```python
from build123d import *

# Parameters (mm, degrees)
F0_W     = 50.8
F0_H     = 50.8
F1_DEPTH = 38.1
F0_H_2   = 12.7
F0_R     = 2.54
F2_DEPTH = 12.7
F3_SIZE  = 5.08
F4_W     = 25.4
F4_H     = 12.7
F5_DEPTH = 38.1


with BuildPart() as f1:
    # F0 (on Top) → F1 (new body)
    with BuildSketch(Plane.XY):
        with Locations((-76.2, 12.7)):
            Rectangle(F0_W, F0_H)
    extrude(amount=F1_DEPTH)

    # F0 (on Top) → F2 (join)
    with BuildSketch(Plane.XY):
        with Locations((-76.2, -19.05)):
            Rectangle(F0_W, F0_H_2)
        with Locations((-95.25, -19.05)):
            Circle(F0_R, mode=Mode.SUBTRACT)
        with Locations((-57.15, -19.05)):
            Circle(F0_R, mode=Mode.SUBTRACT)
        with Locations((-76.2, 44.45)):
            Rectangle(F0_W, F0_H_2)
        with Locations((-95.25, 44.45)):
            Circle(F0_R, mode=Mode.SUBTRACT)
        with Locations((-57.15, 44.45)):
            Circle(F0_R, mode=Mode.SUBTRACT)
    extrude(amount=F2_DEPTH)

    # F3
    f3_edges = [f1.edges().sort_by_distance(p)[0] for p in [
        (-76.2, 38.1, 38.1),
        (-76.2, -12.7, 38.1),
    ]]
    chamfer(f3_edges, length=F3_SIZE)

    # F4 (on face) → F5 (cut)
    with BuildSketch(Plane.YZ.offset(-50.8)):
        with Locations((12.7, 22.86)):
            Rectangle(F4_W, F4_H)
    extrude(amount=-F5_DEPTH, mode=Mode.SUBTRACT)


solid = f1.part
```
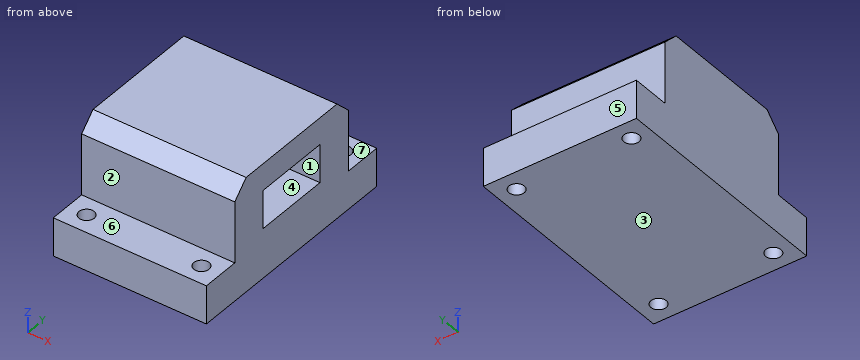
Model file for the job. Use its own axes, mm. Face numbers are marked on the shaded views. A direction names the side the tool comes from. Give positions to 0.01 mm unless a question says otherwise; leave off trailing zeros. Loops run counter-clockwise (first coordinate to the right, second up) from the corner with the lowest first, then second, coordinate; pieces in that order, holes last. Notation, with made-up numbers: (82.25, 48.25) - (125.25, 48.25) arc R21 ccw to (125.25, 65.25) - close; hole circle Ø10 at (-5, 56). An arc over 180 degrees is marked (long way). One line per item, written item: value. Start each with the question number.
1. Which spindle directions (+Z, -Z, +X, -X, +Y, -Y) get a long thin tool onto all of the face, cutting with end or side? Do the marked faces 5, 6 and 7. Say none if no direction does.
2. Probe L1, parallel to Y at x = -95.25, z = 10.25; L2, parallel to X at y = -19, z = 5; L3, parallel to Z at x = -68, y = 11.5. List the from-to ranges inside material, lowest first. Write a range as from..to.
3. Slice it at D-D (x = -80.5). List the corners of the cut face in (y, z).
4. Pin check, flat tips, straight feed: pin 1 (14 mm diameter, centred on x = -69, z = 22, fed in from -Y); pin 2 (4 mm diameter, centred on x = -86.5, y = 42, fed in from +Z); pin 3 (16.5 mm diameter, centred on x = -80, z = 23.5, fed in from +Y). Stop position of each tip, or through.
5. Slice it at C-C (y = 44.45). List the corners of the cut face in (x, z), plus the area to 3 significant figures.
6. Slice it at A-A (x = -95.25). List the corners of the cut face in (y, z).
7. Pull direction Y, two halves, no side cores. Call the marked faces 1, 2, 3 and 4: pulls with the +Y half, pulls with the -Y half, needs draft (parallel to the pull), parting line crosses it, or undercut.
8. Slice it at B-B (z = 3). List the corners of the cut face in (x, y).
Solution:
1. face 5: +Z, -Z, +X, -X, +Y
1. face 6: +Z, +X, -X, -Y
1. face 7: +Z, +X, -X, +Y
2. L1: y = -25.4..-21.59, -16.51..41.91, 46.99..50.8
2. L2: x = -101.6..-97.79, -92.71..-59.69, -54.61..-50.8
2. L3: z = 0..16.51, 29.21..38.1
3. outline: (-25.4, 0) - (50.8, 0) - (50.8, 12.7) - (38.1, 12.7) - (38.1, 33.02) - (33.02, 38.1) - (-7.62, 38.1) - (-12.7, 33.02) - (-12.7, 12.7) - (-25.4, 12.7) - close; hole (0, 16.51) - (25.4, 16.51) - (25.4, 29.21) - (0, 29.21) - close
4. pin 1: stops at y = -12.7
4. pin 2: stops at z = 12.7
4. pin 3: stops at y = 38.1
5. outline: (-101.6, 0) - (-97.79, 0) - (-97.79, 12.7) - (-101.6, 12.7) - close; (-92.71, 0) - (-59.69, 0) - (-59.69, 12.7) - (-92.71, 12.7) - close; (-54.61, 0) - (-50.8, 0) - (-50.8, 12.7) - (-54.61, 12.7) - close
5. area: 516 mm^2
6. outline: (-25.4, 0) - (-21.59, 0) - (-21.59, 12.7) - (-25.4, 12.7) - close; (-16.51, 0) - (41.91, 0) - (41.91, 12.7) - (38.1, 12.7) - (38.1, 33.02) - (33.02, 38.1) - (-7.62, 38.1) - (-12.7, 33.02) - (-12.7, 12.7) - (-16.51, 12.7) - close; (46.99, 0) - (50.8, 0) - (50.8, 12.7) - (46.99, 12.7) - close
7. face 1: undercut
7. face 2: pulls with the -Y half
7. face 3: needs draft
7. face 4: undercut
8. outline: (-101.6, -25.4) - (-50.8, -25.4) - (-50.8, 50.8) - (-101.6, 50.8) - close; hole circle Ø5.08 at (-95.25, -19.05); hole circle Ø5.08 at (-95.25, 44.45); hole circle Ø5.08 at (-57.15, -19.05); hole circle Ø5.08 at (-57.15, 44.45)
